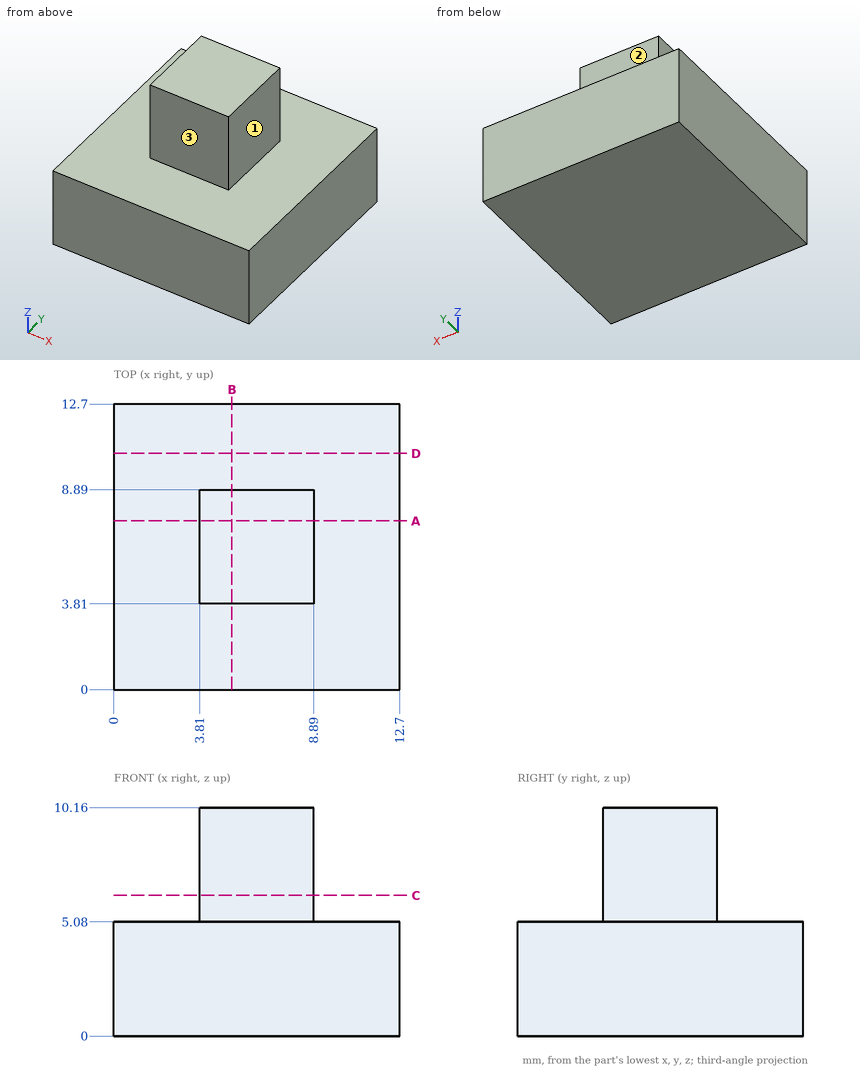
The drawing under review shows one solid part. Ordinate dimensions are in mm from its lowest x, y, z. A direction names the side the tool comes from. Give positions to 0.01 mm unless a question says otherwise; leave off trailing zeros. Write each loop counter-clockwise with the first axis right and the second up, starting at its lowest first coordinate (ties: lowest second). Pieces come first, ordered by that corner, then holes. Notation, with made-up numbers: (55, 89.25) -> (95, 89.25) arc R31 ccw to (95, 124.25) -> close; hole circle Ø1 at (-34.5, 3.25). An arc over 180 degrees is marked (long way). Put each result on its own line as item: value.
(1) Tool access review of the marked faces 1, 2 and 3: name each direction out of +Z, -Z, +X, -X, +Y, -Y from which nothing blocks a thin tool from reaching the whole face with its end or side.
Results are:
face 1: +Z, +X, +Y, -Y
face 2: +Z, +X, -X, +Y
face 3: +Z, +X, -X, -Y
(2) We need section A-A, the plane y = 7.5. Give the boundary of the cut face in (x, z).
Results are:
outline: (0, 0) -> (12.7, 0) -> (12.7, 5.08) -> (8.89, 5.08) -> (8.89, 10.16) -> (3.81, 10.16) -> (3.81, 5.08) -> (0, 5.08) -> close
(3) For pin 1 Ø2.5 at (y, z) = (6, 6.5) entering from -X; pin 2 Ø3 at (x, y) = (1.5, 9) entering from +Z; pin 3 Ø4 at (y, z) = (7.5, 7.5) entering from +X, all flat-tipped, find the tip position at first contact; note any pin that passes through.
Results are:
pin 1: x = 3.81
pin 2: z = 5.08
pin 3: x = 8.89
(4) To check wall thickness, follow probe 1 along Z at (x, y) = (10.25, 4); probe 2 along Y at (x, z) = (8, 7). State the ranges of each line that lie inside material, in increasing order. Write a range as from..to.
Results are:
probe 1: 0..5.08
probe 2: 3.81..8.89
(5) We need section C-C, the plane z = 6.25. Give the boundary of the cut face in (x, y).
Results are:
outline: (3.81, 3.81) -> (8.89, 3.81) -> (8.89, 8.89) -> (3.81, 8.89) -> close
(6) We need section D-D, the plane y = 10.5. Give the boundary of the cut face in (x, z), and give its area (3 significant figures).
Results are:
outline: (0, 0) -> (12.7, 0) -> (12.7, 5.08) -> (0, 5.08) -> close
area: 64.5 mm²
